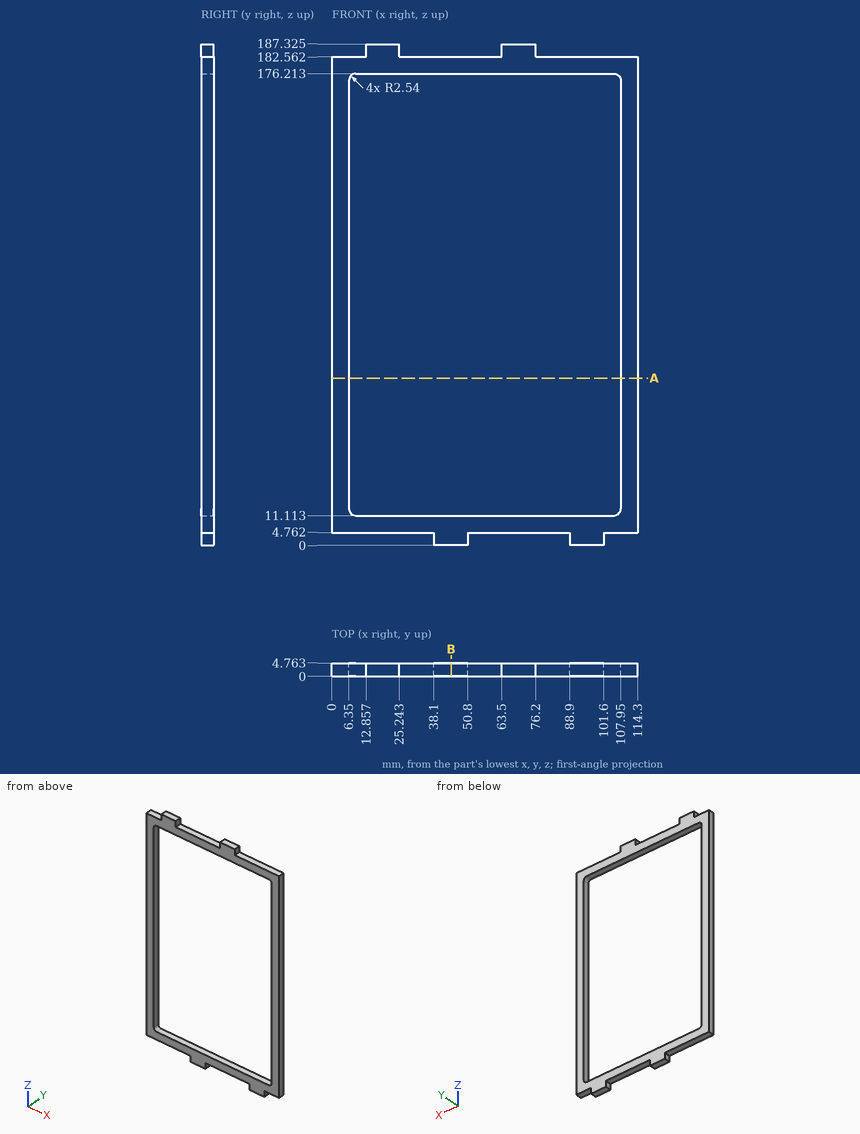
Print and shaded views of the part. All mm, measured from the part's lowest x, y and z. Give positions to 0.01 mm unless a question says otherwise; leave off trailing zeros. Write each loop counter-clockwise with the first axis right and the second up, starting at its lowest first coordinate (ties: lowest second). Pieces come first, ordered by that corner, then holes. Notation, with made-up numbers: (66.5, 33) -> (101.5, 33) arc R20 ccw to (101.5, 42) -> close; hole circle Ø2 at (0, -37). An arc over 180 degrees is marked (long way). Write item = value, one per line.
(1) Slice it at A-A, the plane z = 62.5. Give the cut face in (x, y).
Determined:
outline = (0, 0) -> (6.35, 0) -> (6.35, 4.76) -> (0, 4.76) -> close; (107.95, 0) -> (114.3, 0) -> (114.3, 4.76) -> (107.95, 4.76) -> close
(2) Flat gauge pins, fed straight in: P1, Ø1.4, axis at y = 1.5, z = 184.5, coming from the -X side; P2, Ø1.4, axis at y = 1, z = 3.5, coming from the -X side; P3, Ø1.4, axis at x = 43.5, y = 3.5, coming from the +Z side. Where does each tip first touch, or does it go through?
Determined:
P1 = 12.86
P2 = 38.1
P3 = 182.56
(3) Slice it at B-B, the plane x = 44.5. Give the cut face in (y, z).
Determined:
outline = (0, 0) -> (4.76, 0) -> (4.76, 11.11) -> (0, 11.11) -> close; (0, 176.21) -> (4.76, 176.21) -> (4.76, 182.56) -> (0, 182.56) -> close
(4) Probe line 1 along X through (y, z) = (0.65, 32); line 2 along Z through (x, y) = (94, 3.2); line 3 along Z through (x, y) = (52.5, 1.8). List the from-to ranges inside material, lowest first.
Determined:
line_1 = 0 to 6.35, 107.95 to 114.3
line_2 = 0 to 11.11, 176.21 to 182.56
line_3 = 4.76 to 11.11, 176.21 to 182.56
